The model under review builds one solid part; all positions refer to its coordinate system, in mm. A direction names the side the tool comes from. Coordinates: 2 decimals unless noted, no trailing zeros. Order: outer loops, then holes, each group sorted by start corner. A loop starts at its lowest first (then second) coordinate and runs counter-clockwise, first axis right, second up.
```python
from build123d import *

# Parameters (mm, degrees)
SKETCH1_W                 = 95
SKETCH1_H                 = 90
BOSS_EXTRUDE1_DEPTH       = 25.1
SHELL1_T                  = -7.82
SHELL1_THICKNESS_2_FACE_W = 79.36
SHELL1_THICKNESS_2_FACE_H = 74.36
SHELL1_THICKNESS_2_DEPTH  = 2.97


with BuildPart() as part:
    # Sketch1 → Boss-Extrude1 (new body)
    with BuildSketch(Plane.XY):
        Rectangle(SKETCH1_W, SKETCH1_H)
    extrude(amount=BOSS_EXTRUDE1_DEPTH)

    # Shell1
    shell1_openings = [part.faces().sort_by_distance(p)[0] for p in [
        (0, 0, 0),
    ]]
    offset(amount=SHELL1_T, openings=shell1_openings, kind=Kind.INTERSECTION)

    # Shell1 thickness 2 face (on inner face of the shell) → Shell1 thickness 2 (add)
    with BuildSketch(Plane.XY.offset(17.28)):
        Rectangle(SHELL1_THICKNESS_2_FACE_W, SHELL1_THICKNESS_2_FACE_H)
    extrude(amount=-SHELL1_THICKNESS_2_DEPTH)


solid = part.part
```
(1) Draft analysis for pull direction X (two halves, no side actions). For faces 1 (the face through (47.5, -1, 12)), 2 (the face through (-1, 37.18, 7)), 3 (the face through (-1, 1, 14.31)), 4 (the face through (-47.5, -1, 12)), state which applies: released by +X, released by -X, zero draft, split by the parting line, or undercut.
A:
face 1: released by +X
face 2: undercut
face 3: undercut
face 4: released by -X
(2) We need section B-B, the plane x = 9. Write out the cut boundary in (y, z).
A:
outline: (-45, 0) - (-37.18, 0) - (-37.18, 14.31) - (37.18, 14.31) - (37.18, 0) - (45, 0) - (45, 25.1) - (-45, 25.1) - close
(3) We need section C-C, the plane y = 13.5. Write out the cut boundary in (x, z).
A:
outline: (-47.5, 0) - (-39.68, 0) - (-39.68, 14.31) - (39.68, 14.31) - (39.68, 0) - (47.5, 0) - (47.5, 25.1) - (-47.5, 25.1) - close
(4) Wall thickness on probe 1 along X at (y, z) = (12, 6.75); probe 2 along Y at (x, z) = (-39, 9); probe 3 along Z at (x, y) = (6.5, 37): over which ranges is each line inside the solid? List them lowest first.
A:
probe 1: x = -47.5 to -39.68, 39.68 to 47.5
probe 2: y = -45 to -37.18, 37.18 to 45
probe 3: z = 14.31 to 25.1
(5) For pin 1 Ø22.5 at (x, y) = (-16, 14.5) entering from -Z, flat-tipped, find the tip position at first contact; note if it passes through.
A:
pin 1: stops at z = 14.31
(6) We need section A-A, the plane z = 2. Write out the cut boundary in (x, y).
A:
outline: (-47.5, -45) - (47.5, -45) - (47.5, 45) - (-47.5, 45) - close; hole (-39.68, -37.18) - (39.68, -37.18) - (39.68, 37.18) - (-39.68, 37.18) - close
(7) Machinability: for faces 5 (the face through (-39.68, -1, 7)), 6 (the face through (-1, -39, 0)), which of the approach directions +Z, -Z, +X, -X, +Y, -Y give a long, thin tool a straight path to every point of the face, cutting with its end or side? Answer none if there is none.
A:
face 5: -Z
face 6: -Z, +X, -X, +Y, -Y
